Check sheet for the drawn part. Datum: minimum x, y, z corner. Units: mm. Coordinates: 2 decimals unless noted, no trailing zeros. Loops run counter-clockwise (first coordinate to the right, second up) from the corner with the lowest first, then second, coordinate; pieces in that order, holes last.
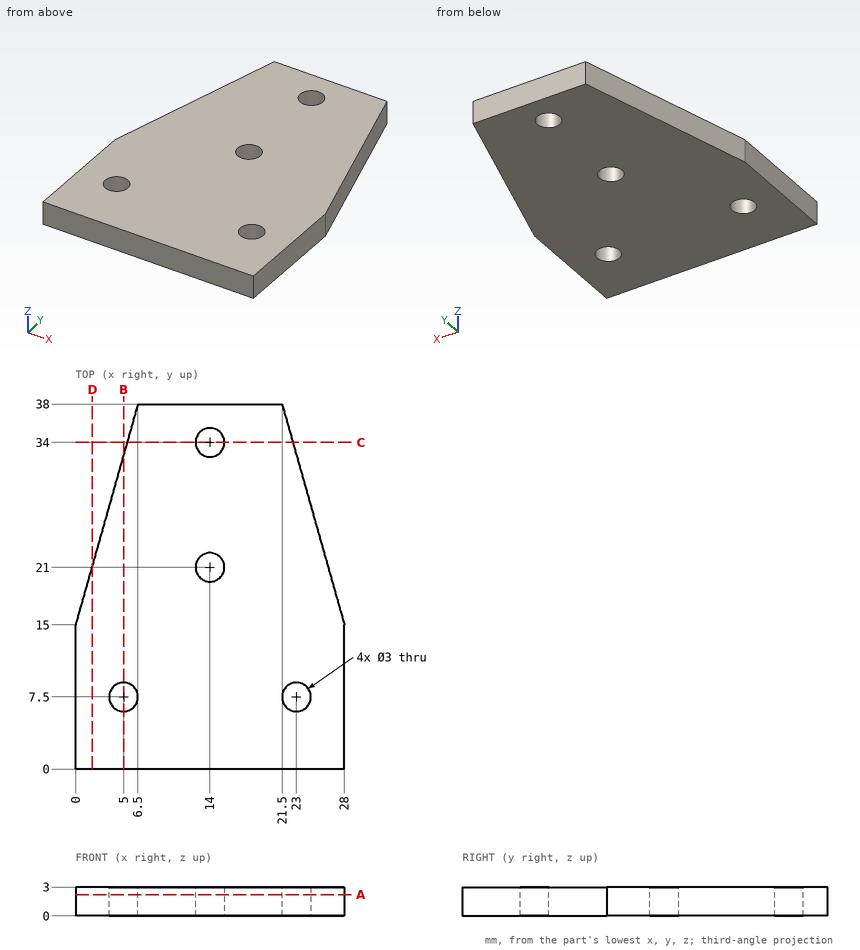
1) Scan lines: line 1 (Y direction, x = 14, z = 0.7); line 2 (X direction, y = 8.5, z = 2.35); line 3 (X direction, y = 28.5, z = 2.6). Record each from-to range of solid material in increasing order.
Answer sheet:
line 1: y = 0 to 19.5, 22.5 to 32.5, 35.5 to 38
line 2: x = 0 to 3.88, 6.12 to 21.88, 24.12 to 28
line 3: x = 3.82 to 24.18
2) Section check B-B on x = 5. Enter the section's corners in (y, z), plus the area to 3 significant figures.
Answer sheet:
outline: (0, 0) - (6, 0) - (6, 3) - (0, 3) - close; (9, 0) - (32.69, 0) - (32.69, 3) - (9, 3) - close
area: 89.1 mm2
3) Section check C-C on y = 34. Enter the section's corners in (x, z), plus the area to 3 significant figures.
Answer sheet:
outline: (5.37, 0) - (12.5, 0) - (12.5, 3) - (5.37, 3) - close; (15.5, 0) - (22.63, 0) - (22.63, 3) - (15.5, 3) - close
area: 42.8 mm2
4) Section check A-A on z = 2.2. Enter the section's corners in (x, y), plus the area to 3 significant figures.
Answer sheet:
outline: (0, 0) - (28, 0) - (28, 15) - (21.5, 38) - (6.5, 38) - (0, 15) - close; hole circle Ø3 at (5, 7.5); hole circle Ø3 at (14, 21); hole circle Ø3 at (14, 34); hole circle Ø3 at (23, 7.5)
area: 886 mm2
5) Depth check by flat-ended pin: pin 1 (1 mm diameter, centred on y = 28.5, z = 0.5, fed in from -X). Enter the tip coordinate at first touch or a pass-through.
Answer sheet:
pin 1: stops at x = 3.67
6) Section check D-D on x = 1.75. Enter the section's corners in (y, z), plus the area to 3 significant figures.
Answer sheet:
outline: (0, 0) - (21.19, 0) - (21.19, 3) - (0, 3) - close
area: 63.6 mm2
